from build123d import *

# Parameters (mm, degrees)
SKETCH1_W           = 57.15
SKETCH1_H           = 63.5
BOSS_EXTRUDE1_DEPTH = 120
SKETCH2_W           = 21.25
SKETCH2_H           = 41.25
CUT_EXTRUDE1_DEPTH  = 25
SKETCH3_R           = 2.2
CUT_EXTRUDE2_DEPTH  = 10
SKETCH4_W           = 21.25
SKETCH4_H           = 15
CUT_EXTRUDE3_DEPTH  = 64.5
SKETCH7_R           = 2.05
CUT_EXTRUDE4_DEPTH  = 58.15
SKETCH9_W           = 12
SKETCH9_H           = 7
BOSS_EXTRUDE2_DEPTH = 57.15
SKETCH10_R          = 2.05
CUT_EXTRUDE5_DEPTH  = 8
BOSS_EXTRUDE3_DEPTH = 7
BOSS_EXTRUDE4_DEPTH = 7
SKETCH13_W          = 21.25
SKETCH13_H          = 20
CUT_EXTRUDE6_DEPTH  = 60


with BuildPart() as part:
    # Sketch1 → Boss-Extrude1 (new body)
    with BuildSketch(Plane(origin=(0, 0, 0), x_dir=(1, 0, 0), z_dir=(0, 1, 0))):
        Rectangle(SKETCH1_W, SKETCH1_H)
    extrude(amount=BOSS_EXTRUDE1_DEPTH)

    # Sketch2 → Cut-Extrude1 (cut)
    with BuildSketch(Plane(origin=(0, 120, 0), x_dir=(1, 0, 0), z_dir=(0, 1, 0))):
        Rectangle(SKETCH2_W, SKETCH2_H)
    extrude(amount=-CUT_EXTRUDE1_DEPTH, mode=Mode.SUBTRACT)

    # Sketch3 → Cut-Extrude2 (cut)
    with BuildSketch(Plane(origin=(0, 120, 0), x_dir=(1, 0, 0), z_dir=(0, 1, 0))):
        with Locations((5.325, 24.725)):
            Circle(SKETCH3_R)
        with Locations((-5.325, 24.725)):
            Circle(SKETCH3_R)
        with Locations((5.325, -24.725)):
            Circle(SKETCH3_R)
        with Locations((-5.325, -24.725)):
            Circle(SKETCH3_R)
    extrude(amount=-CUT_EXTRUDE2_DEPTH, mode=Mode.SUBTRACT)

    # Sketch4 → Cut-Extrude3 (cut, through all)
    with BuildSketch(Plane.XY.offset(31.75)):
        with Locations((0, 106.5)):
            Rectangle(SKETCH4_W, SKETCH4_H)
    extrude(amount=-CUT_EXTRUDE3_DEPTH, mode=Mode.SUBTRACT)

    # Sketch7 → Cut-Extrude4 (cut, through all)
    with BuildSketch(Plane.ZY.offset(28.575)):
        with Locations((23.75, 20)):
            Circle(SKETCH7_R)
        with Locations((23.75, 90)):
            Circle(SKETCH7_R)
        with Locations((-23.75, 20)):
            Circle(SKETCH7_R)
        with Locations((-23.75, 90)):
            Circle(SKETCH7_R)
    extrude(amount=-CUT_EXTRUDE4_DEPTH, mode=Mode.SUBTRACT)

    # Sketch9 → Boss-Extrude2 (add)
    with BuildSketch(Plane(origin=(28.575, 0, 0), x_dir=(0, 0, -1), z_dir=(1, 0, 0))):
        with Locations((37.75, 3.5)):
            Rectangle(SKETCH9_W, SKETCH9_H)
        with Locations((-37.75, 3.5)):
            Rectangle(SKETCH9_W, SKETCH9_H)
    extrude(amount=-BOSS_EXTRUDE2_DEPTH)

    # Sketch10 → Cut-Extrude5 (cut, through all)
    with BuildSketch(Plane(origin=(0, 7, 0), x_dir=(1, 0, 0), z_dir=(0, 1, 0))):
        with Locations((-14.575, 37.75)):
            Circle(SKETCH10_R)
        with Locations((14.575, 37.75)):
            Circle(SKETCH10_R)
        with Locations((14.575, -37.75)):
            Circle(SKETCH10_R)
        with Locations((-14.575, -37.75)):
            Circle(SKETCH10_R)
    extrude(amount=-CUT_EXTRUDE5_DEPTH, mode=Mode.SUBTRACT)

    # Sketch11 → Boss-Extrude3 (add)
    with BuildSketch(Plane(origin=(28.575, 0, 0), x_dir=(0, 0, -1), z_dir=(1, 0, 0))):
        Polygon((-31.75, 45.157568057), (-43.75, 7), (-31.75, 7), align=None)
        Polygon((43.75, 7), (31.75, 7), (31.75, 45.157568057), align=None)
    extrude(amount=-BOSS_EXTRUDE3_DEPTH)

    # Sketch12 → Boss-Extrude4 (add)
    with BuildSketch(Plane.ZY.offset(28.575)):
        Polygon((-31.75, 45.157568057), (-43.75, 7), (-31.75, 7), align=None)
        Polygon((43.75, 7), (31.75, 7), (31.75, 45.157568057), align=None)
    extrude(amount=-BOSS_EXTRUDE4_DEPTH)

    # Sketch13 → Cut-Extrude6 (cut)
    with BuildSketch(Plane(origin=(0, 95, 0), x_dir=(1, 0, 0), z_dir=(0, 1, 0))):
        Rectangle(SKETCH13_W, SKETCH13_H)
    extrude(amount=-CUT_EXTRUDE6_DEPTH, mode=Mode.SUBTRACT)


solid = part.part
Geometry check sheet. Reference: the model listing, model coordinates, mm. A direction names the side the tool comes from. Give positions to 0.01 mm unless a question says otherwise; leave off trailing zeros. Write each loop counter-clockwise with the first axis right and the second up, starting at its lowest first coordinate (ties: lowest second). Pieces come first, ordered by that corner, then holes.
1) Thickness scan on line 1 (X direction, y = 62.5, z = -1) (3 decimals); line 2 (X direction, y = 5, z = 37) (3 decimals); line 3 (Z direction, x = 19, y = 25). Record the ranges inside material, lowest first.
Values follow:
line 1: x = -28.575 to -10.625, 10.625 to 28.575
line 2: x = -28.575 to -16.483, -12.667 to 12.667, 16.483 to 28.575
line 3: z = -31.75 to 31.75
2) Release check for a two-part mould opening along Z. For faces 1 (the face through (0, 114, -26)), 2 (the face through (-14.842, 3.549, 35.717)), 3 (the face through (25.124, 26.346, 37.666)) record: released by +Z, released by -Z, zero draft, split by the parting line, or undercut.
Values follow:
face 1: zero draft
face 2: undercut
face 3: released by +Z
3) Go/stop test with flat-tipped pins: pin 1 Ø5 at (x, y) = (1.5, 118) entering from -Z; pin 2 Ø1.5 at (x, y) = (21, 70.5) entering from +Z; pin 3 Ø5 at (x, z) = (-18.5, -23.5) entering from -Y; pin 4 Ø3.5 at (y, z) = (90, 23.75) entering from -X. Record where each tip stops, or that it passes through.
Values follow:
pin 1: stops at z = -31.75
pin 2: stops at z = 31.75
pin 3: stops at y = 0
pin 4: passes through
4) Cross-section at C-C (z = -30). Record the boundary of the cut face in (x, y) (3 decimals).
Values follow:
outline: (-28.575, 0) - (28.575, 0) - (28.575, 120) - (-28.575, 120) - close; hole (-10.625, 99) - (10.625, 99) - (10.625, 114) - (-10.625, 114) - close
5) Cross-section at A-A (y = 103.5). Record the boundary of the cut face in (x, z) (3 decimals).
Values follow:
outline: (-28.575, -31.75) - (-10.625, -31.75) - (-10.625, 31.75) - (-28.575, 31.75) - close; (10.625, -31.75) - (28.575, -31.75) - (28.575, 31.75) - (10.625, 31.75) - close
6) Cross-section at D-D (y = 47.5). Record the boundary of the cut face in (x, z) (3 decimals).
Values follow:
outline: (-28.575, -31.75) - (28.575, -31.75) - (28.575, 31.75) - (-28.575, 31.75) - close; hole (-10.625, -10) - (10.625, -10) - (10.625, 10) - (-10.625, 10) - close
7) Cross-section at B-B (x = 19.5). Record the boundary of the cut face in (y, z).
Values follow:
outline: (0, -43.75) - (7, -43.75) - (7, -31.75) - (120, -31.75) - (120, 31.75) - (7, 31.75) - (7, 43.75) - (0, 43.75) - close; hole circle Ø4.1 at (20, -23.75); hole circle Ø4.1 at (20, 23.75); hole circle Ø4.1 at (90, -23.75); hole circle Ø4.1 at (90, 23.75)
8) Set-up check for faces 4 (the face through (0, 65, 10)), 5 (the face through (0, 99, 26)), 6 (the face through (0, 7, -38)), 7 (the face through (-28.575, 61, -1)), 8 (the face through (-21.575, 18, 35)): record each of +Z, -Z, +X, -X, +Y, -Y from which the full face is reachable in a straight line by a thin tool's end or side.
Values follow:
face 4: +Y
face 5: +Z, -Z
face 6: -Z, +Y
face 7: +Z, -Z, -X, +Y, -Y
face 8: +Z, +Y
